Job drawing, mm, ordinate dimensions from the low corner. One solid piece. Round coordinates to 2 decimals unless told otherwise and drop trailing zeros. Loops run counter-clockwise (first coordinate to the right, second up) from the corner with the lowest first, then second, coordinate; pieces in that order, holes last. Notation, with made-up numbers: (47, 41) - (90, 41) arc R25 cw to (90, 62) - close; hole circle Ø1 at (9.25, 52). An arc over 180 degrees is marked (long way). Answer as CSV lines item,"result". Start each with the question number.
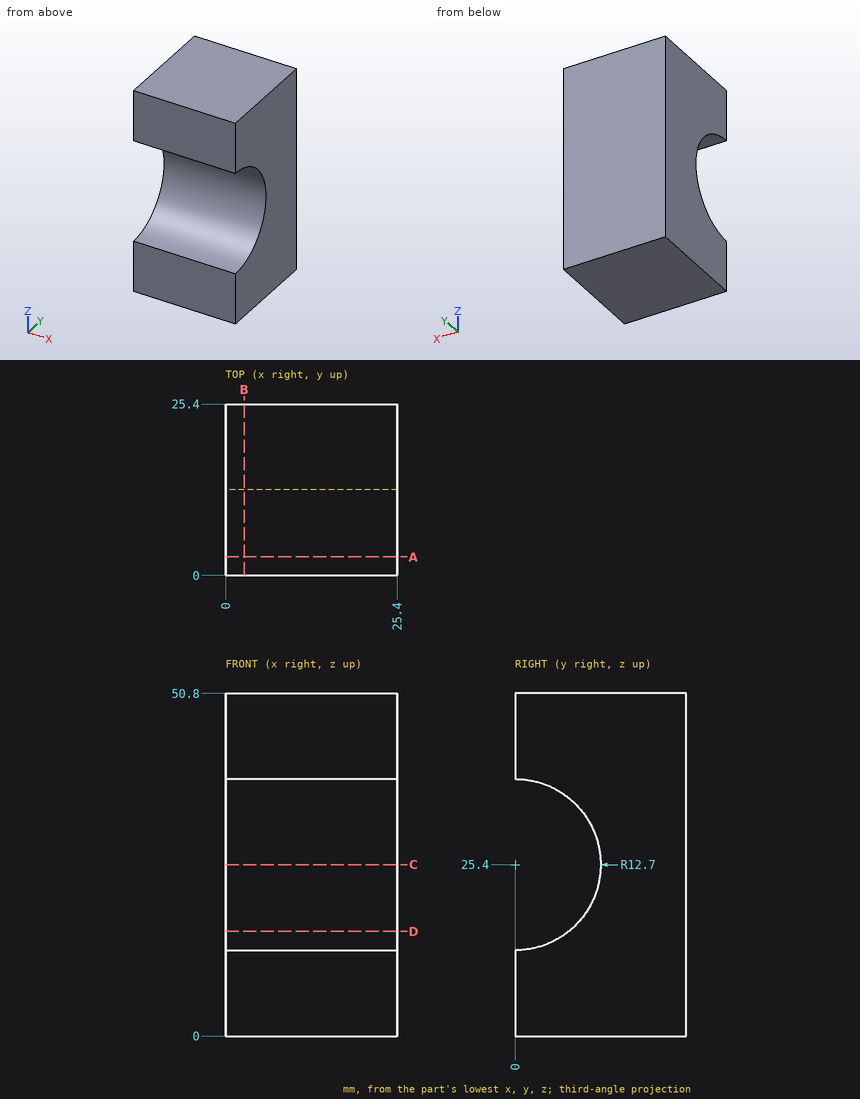
Q1. Pin check, flat tip, straight feed: pin 1 Ø10 at (y, z) = (5.5, 36.5) entering from +X. Stop position of the tip, or through.
Q2. Wall check: probe 1 along Z at (x, y) = (2.5, 7.5); probe 2 along Z at (x, y) = (3.75, 8.75); probe 3 along Y at (x, z) = (10.25, 29). Give the ranges that are in metal, low to high. Write a range as [from, to].
Q3. Band-saw the part on B-B, the plane x = 2.75. List the corners of the cut face in (y, z).
Q4. Band-saw the part on C-C, the plane z = 25.4. List the corners of the cut face in (x, y).
Q5. Band-saw the part on A-A, the plane y = 2.75. List the corners of the cut face in (x, z).
Q6. Band-saw the part on D-D, the plane z = 15.5. List the corners of the cut face in (x, y).
Reported:
1,pin 1,"stops at x = 25.4"
2,probe 1,"z = [0, 15.15], [35.65, 50.8]"
2,probe 2,"z = [0, 16.2], [34.6, 50.8]"
2,probe 3,"y = [12.18, 25.4]"
3,outline,"(0, 0) - (25.4, 0) - (25.4, 50.8) - (0, 50.8) - (0, 38.1) arc R12.7 cw to (0, 12.7) - close"
4,outline,"(0, 12.7) - (25.4, 12.7) - (25.4, 25.4) - (0, 25.4) - close"
5,outline,"(0, 0) - (25.4, 0) - (25.4, 13) - (0, 13) - close; (0, 37.8) - (25.4, 37.8) - (25.4, 50.8) - (0, 50.8) - close"
6,outline,"(0, 7.95) - (25.4, 7.95) - (25.4, 25.4) - (0, 25.4) - close"
